Source: CAD feature listing. Evaluate the final solid. Frame: model axes, mm. A direction names the side the tool comes from. Give positions to 0.01 mm unless a question says otherwise; leave off trailing zeros. Write each loop counter-clockwise with the first axis right and the second up, starting at its lowest first coordinate (ties: lowest second). Pieces come first, ordered by that corner, then holes. Notation, with made-up numbers: (-23, -0.75) -> (0, -0.75) arc R36 cw to (0, 34.25) -> close; hole circle Ø8 at (13, 3.5). An arc over 180 degrees is marked (long way). Use one line per item in the form item = value. Start each with the question number.
(1) First-contact query: P1, Ø3.5, axis at y = 26, z = -17, coming from the +X side; P2, Ø6, axis at x = 53, y = 9, coming from the -Z side; P3, Ø8, axis at x = 40.5, z = -19.5, coming from the -Y side; P4, Ø10, axis at y = 24.5, z = -14, coming from the -X side. Flat tips, straight axial feed; report the tip coordinate or a pass-through.
(2) Material intervals for line 1 along X through (y, z) = (4.75, 2.5); line 2 along X through (y, z) = (25.9, -18); line 3 along Z through (x, y) = (144, 4.75), sorted ascending. Write a range as from..to.
(3) Set-up query: faces 1 (the face through (207, 1, -10)), 2 (the face through (141, 10, -14)), 3 (the face through (17.833, 9.727, -6.902)), 4 (the face through (101, 1, 3)). Return all of +Z, -Z, +X, -X, +Y, -Y with unobstructed straight access to the full face (end or side cutting, diameter ignored); none if empty.
(4) Cut plane A-A, the plane y = 21.25. Output: boundary loops of the cut face in (x, z).
from build123d import *

# Parameters (mm, degrees)
BLANKSKE_W          = 209
BLANKSKE_H          = 12.5
BLANK_DEPTH         = 14
TOOTHCUTSIM_DEPTH   = 210.841011244
TEETHCUTS_COUNT     = 27
TEETHCUTS_PITCH     = 7.853981625
SKETCH2_W           = 110
SKETCH2_H           = 6.78
BOSS_EXTRUDE2_DEPTH = 7
SKETCH3_W           = 110
SKETCH3_H           = 56
BOSS_EXTRUDE3_DEPTH = 5
SKETCH4_W           = 110
SKETCH4_H           = 6.78
BOSS_EXTRUDE4_DEPTH = 7
SKETCH7_W           = 110
SKETCH7_H           = 6.78
BOSS_EXTRUDE5_DEPTH = 6
SKETCH8_W           = 110
SKETCH8_H           = 6.78
BOSS_EXTRUDE6_DEPTH = 20
SKETCH9_W           = 110
SKETCH9_H           = 7
BOSS_EXTRUDE7_DEPTH = 5.72
SKETCH5_R           = 1.5
CUT_EXTRUDE1_DEPTH  = 218.928887484
SKETCH6_R           = 1.5
CUT_EXTRUDE2_DEPTH  = 219.050452877
FILLET1_R           = 5
SKETCH12_W          = 119.263366365
SKETCH12_H          = 39.167998327
CUT_EXTRUDE3_DEPTH  = 28
SKETCH13_W          = 6
SKETCH13_H          = 3
BOSS_EXTRUDE8_DEPTH = 6
SKETCH14_R          = 1.5
CUT_EXTRUDE4_DEPTH  = 6


with BuildPart() as part:
    # BlankSke → Blank (new body)
    with BuildSketch(Plane.XY):
        with Locations((104.5, 6.25)):
            Rectangle(BLANKSKE_W, BLANKSKE_H)
    extrude(amount=-BLANK_DEPTH)

    # TooCutSkeSim → ToothCutSim (cut, through all)
    with BuildSketch(Plane.XY):
        Polygon((1.087088424, 6.875), (-1.087088424, 6.875), (-3.143665836, 12.5254), (3.143665836, 12.5254), align=None)
    toothcutsim = extrude(amount=-TOOTHCUTSIM_DEPTH, mode=Mode.SUBTRACT)

    # TeethCuts: ToothCutSim ×27
    with Locations(*[(i * TEETHCUTS_PITCH, 0, 0) for i in range(1, TEETHCUTS_COUNT)]):
        add(toothcutsim, mode=Mode.SUBTRACT)

    # Sketch2 → Boss-Extrude2 (add)
    with BuildSketch(Plane(origin=(0, 0, -14), x_dir=(-1, 0, 0), z_dir=(0, 0, -1))):
        with Locations((-154, 3.39)):
            Rectangle(SKETCH2_W, SKETCH2_H)
    extrude(amount=BOSS_EXTRUDE2_DEPTH)

    # Sketch3 → Boss-Extrude3 (add)
    with BuildSketch(Plane(origin=(0, 0, -21), x_dir=(-1, 0, 0), z_dir=(0, 0, -1))):
        with Locations((-154, 28)):
            Rectangle(SKETCH3_W, SKETCH3_H)
    extrude(amount=BOSS_EXTRUDE3_DEPTH)

    # Sketch4 → Boss-Extrude4 (add)
    with BuildSketch(Plane.XY.offset(-21)):
        with Locations((154, 52.61)):
            Rectangle(SKETCH4_W, SKETCH4_H)
    extrude(amount=BOSS_EXTRUDE4_DEPTH)

    # Sketch7 → Boss-Extrude5 (add)
    with BuildSketch(Plane.XY):
        with Locations((154, 3.39)):
            Rectangle(SKETCH7_W, SKETCH7_H)
    extrude(amount=BOSS_EXTRUDE5_DEPTH)

    # Sketch8 → Boss-Extrude6 (add)
    with BuildSketch(Plane.XY.offset(-14)):
        with Locations((154, 52.61)):
            Rectangle(SKETCH8_W, SKETCH8_H)
    extrude(amount=BOSS_EXTRUDE6_DEPTH)

    # Sketch9 → Boss-Extrude7 (add)
    with BuildSketch(Plane(origin=(0, 6.78, 0), x_dir=(1, 0, 0), z_dir=(0, 1, 0))):
        with Locations((154, 17.5)):
            Rectangle(SKETCH9_W, SKETCH9_H)
    extrude(amount=BOSS_EXTRUDE7_DEPTH)

    # Sketch5 → Cut-Extrude1 (cut, through all)
    with BuildSketch(Plane.XZ):
        with Locations(Location((164, -17.5, 0), (0, 0, 270))):
            Circle(SKETCH5_R)
        with Locations(Location((144, -17.5, 0), (0, 0, 270))):
            Circle(SKETCH5_R)
        with Locations(Location((144, 2.5, 0), (0, 0, 270))):
            Circle(SKETCH5_R)
        with Locations(Location((164, 2.5, 0), (0, 0, 270))):
            Circle(SKETCH5_R)
    extrude(amount=-CUT_EXTRUDE1_DEPTH, mode=Mode.SUBTRACT)

    # Sketch6 → Cut-Extrude2 (cut, through all)
    with BuildSketch(Plane.XY.offset(-21)):
        with Locations((112.16, 15.28)):
            Circle(SKETCH6_R)
        with Locations((152.16, 15.28)):
            Circle(SKETCH6_R)
        with Locations((192.16, 15.28)):
            Circle(SKETCH6_R)
        with Locations((112.16, 45.28)):
            Circle(SKETCH6_R)
        with Locations((192.16, 45.28)):
            Circle(SKETCH6_R)
        with Locations((152.16, 45.28)):
            Circle(SKETCH6_R)
    extrude(amount=-CUT_EXTRUDE2_DEPTH, mode=Mode.SUBTRACT)

    # Fillet1
    fillet1_edges = [part.edges().sort_by_distance(p)[0] for p in [
        (99, 0, -20),
        (209, 56, -10),
        (99, 56, -10),
        (99, 0, 3),
        (209, 0, -10),
    ]]
    fillet(fillet1_edges, radius=FILLET1_R)

    # Sketch12 → Cut-Extrude3 (cut)
    with BuildSketch(Plane(origin=(0, 56, 0), x_dir=(1, 0, 0), z_dir=(0, 1, 0))):
        with Locations((155.252120093, 7.537257659)):
            Rectangle(SKETCH12_W, SKETCH12_H)
    extrude(amount=-CUT_EXTRUDE3_DEPTH, mode=Mode.SUBTRACT)

    # Sketch13 → Boss-Extrude8 (add)
    with BuildSketch(Plane.XY.offset(-21)):
        with Locations((176, 26.5)):
            Rectangle(SKETCH13_W, SKETCH13_H)
        with Locations((132, 26.5)):
            Rectangle(SKETCH13_W, SKETCH13_H)
    extrude(amount=BOSS_EXTRUDE8_DEPTH)

    # Sketch14 → Cut-Extrude4 (cut)
    with BuildSketch(Plane(origin=(0, 28, 0), x_dir=(-1, 0, 0), z_dir=(0, 1, 0))):
        with Locations(Location((-132, -18, 0), (0, 0, 90))):
            Circle(SKETCH14_R)
        with Locations(Location((-176, -18, 0), (0, 0, 90))):
            Circle(SKETCH14_R)
    extrude(amount=-CUT_EXTRUDE4_DEPTH, mode=Mode.SUBTRACT)


solid = part.part
Geometry says:
q1.P1 = 179
q1.P2 = -14
q1.P3 = through
q1.P4 = 129
q2.line_1 = 99.01..142.5, 145.5..162.5, 165.5..208.99
q2.line_2 = 129..130.5, 133.5..135, 173..174.5, 177.5..179
q2.line_3 = -26..-19, -16..1, 4..6
q3.face_1 = +Z, -Z, +X, -Y
q3.face_2 = +Z, +Y
q3.face_3 = +Z, -Z, +Y
q3.face_4 = +Z, -X, -Y
q4.outline = (99, -26) -> (209, -26) -> (209, -21) -> (99, -21) -> close
